from build123d import *

# Parameters (mm, degrees)
SKETCH1_R           = 3.925
BOSS_EXTRUDE1_DEPTH = 11
SKETCH2_R           = 5.084149635
BOSS_EXTRUDE2_DEPTH = 1.4
SKETCH3_R           = 2.4
CUT_EXTRUDE1_DEPTH  = 15.333776719
CHAMFER1_SIZE       = 0.25
CUT_EXTRUDE2_START  = -6
SKETCH4_R           = 6.115916059
CUT_EXTRUDE2_DEPTH  = 6


with BuildPart() as part:
    # Sketch1 → Boss-Extrude1 (new body)
    with BuildSketch(Plane.XY):
        Circle(SKETCH1_R)
    extrude(amount=-BOSS_EXTRUDE1_DEPTH)

    # Sketch2 → Boss-Extrude2 (add)
    with BuildSketch(Plane.XY):
        Circle(SKETCH2_R)
    extrude(amount=BOSS_EXTRUDE2_DEPTH)

    # Sketch3 → Cut-Extrude1 (cut, through all)
    with BuildSketch(Plane.XY.offset(1.4)):
        Circle(SKETCH3_R)
    extrude(amount=-CUT_EXTRUDE1_DEPTH, mode=Mode.SUBTRACT)

    # Chamfer1
    chamfer1_edges = [part.edges().sort_by_distance(p)[0] for p in [
        (-2.4, 0, -11),
        (-2.4, 0, 1.4),
        (-3.925, 0, -11),
        (-5.084149635, 0, 0),
        (-5.084149635, 0, 1.4),
    ]]
    chamfer(chamfer1_edges, length=CHAMFER1_SIZE)

    # Sketch4 → Cut-Extrude2 (cut)
    with BuildSketch(Plane(origin=(0, 0, -11), x_dir=(-1, 0, 0), z_dir=(0, 0, -1)).offset(CUT_EXTRUDE2_START)):
        Circle(SKETCH4_R)
    extrude(amount=CUT_EXTRUDE2_DEPTH, mode=Mode.SUBTRACT)


solid = part.part
Could you check a few things on this model? Use its own coordinates, in mm. Coordinates: 2 decimals unless noted, no trailing zeros. Write each loop counter-clockwise with the first axis right and the second up, starting at its lowest first coordinate (ties: lowest second). Pieces come first, ordered by that corner, then holes. Notation, with made-up numbers: (-36.5, 20) - (-17.5, 20) arc R11 ccw to (-17.5, 36) - close; hole circle Ø1 at (12, 12). An arc over 180 degrees is marked (long way). Put each result on its own line as item: value. Start each with the question number.
Q1. Thinking about a two-plate mould opening in X: for faces 1 (the flat face through (-1, 4, 0)), 2 (the cylindrical face through (-2.893, 2.653, -2.465)), 3 (the cylindrical face through (1.29, 2.024, -1.882)), which applies, pulls with the +X half, pulls with the -X half, needs draft (parallel to the pull), parting line crosses it, or undercut?
Q2. I want a section at A-A on y = 0. Write out the boundary of the cut face in (x, z) (3 decimals), plus the area to 3 significant figures.
Q3. Please list where these lines run through material, in increasing order: L1, parallel to Y at x = 0, z = -1.75 (3 decimals); L2, parallel to Z at x = 0.5, y = 4.25; L3, parallel to Y at x = -1.5, z = -1.75.
Q4. I want a section at C-C on z = -4. Write out the boundary of the cut face in (x, y) (3 decimals).
Q5. I'm going to push flat-ended pins straight in: P1, Ø3, axis at x = -2, z = 0.5, coming from the -Y side; P2, Ø2, axis at x = -2, z = -2, coming from the +Y side. Where does each tip first touch, or does it pass through?
Checks:
1. face 1: needs draft
1. face 2: parting line crosses it
1. face 3: undercut
2. outline: (-5.084, 0.25) - (-4.834, 0) - (-3.925, 0) - (-3.925, -5) - (-2.4, -5) - (-2.4, 1.15) - (-2.65, 1.4) - (-4.834, 1.4) - (-5.084, 1.15) - close; (2.4, -5) - (3.925, -5) - (3.925, 0) - (4.834, 0) - (5.084, 0.25) - (5.084, 1.15) - (4.834, 1.4) - (2.65, 1.4) - (2.4, 1.15) - close
2. area: 22.6 mm²
3. L1: -3.925 to -2.4, 2.4 to 3.925
3. L2: 0 to 1.4
3. L3: -3.63 to -1.87, 1.87 to 3.63
4. outline: circle Ø7.85 at (0, 0); hole circle Ø4.8 at (0, 0)
5. P1: y = -5.06
5. P2: y = 3.8
